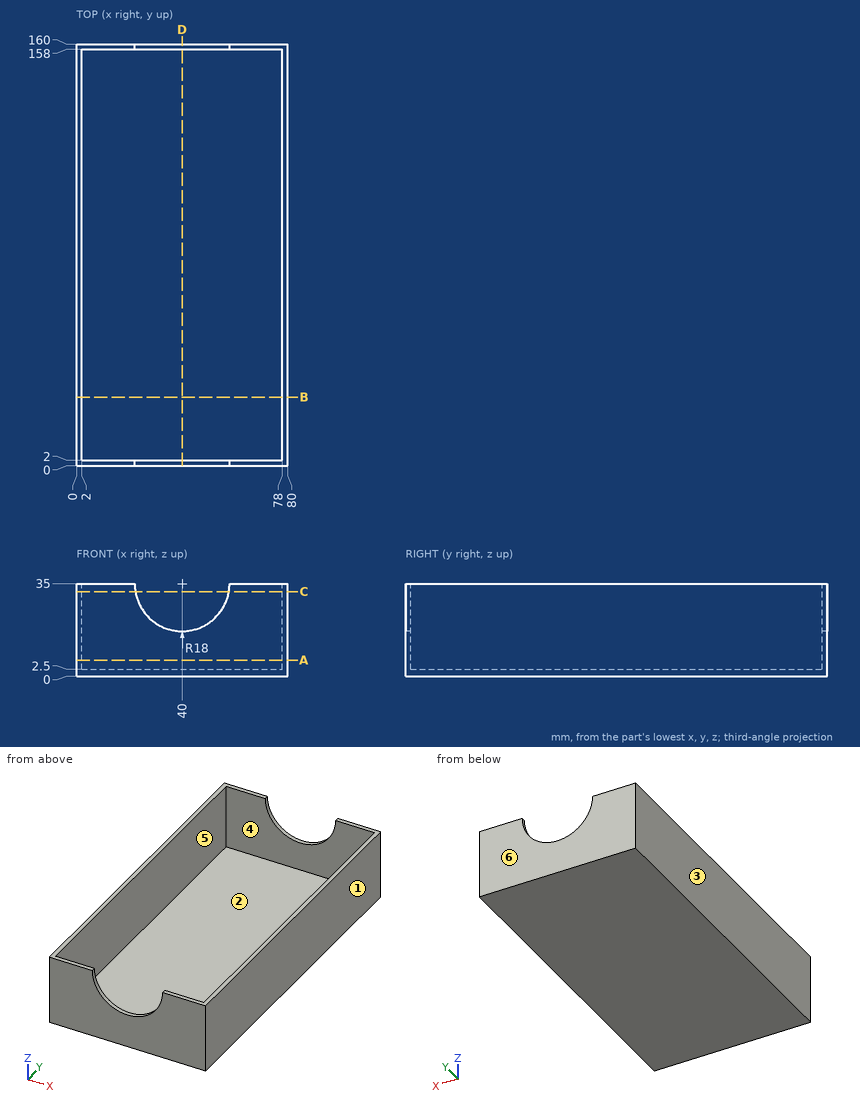
Input: dimensioned drawing with shaded views. Units: mm. Origin: part minimum x, y, z. A direction names the side the tool comes from. Round coordinates to 2 decimals unless told otherwise and drop trailing zeros. Loops run counter-clockwise (first coordinate to the right, second up) from the corner with the lowest first, then second, coordinate; pieces in that order, holes last. Notation, with made-up numbers: (52.25, 4.5) -> (57.25, 4.5) arc R25 cw to (57.25, 39.5) -> close; hole circle Ø8 at (13, 48). An arc over 180 degrees is marked (long way). Answer as a JSON object with one key per item and string values. Group by question number.
Q1. Section query C-C (z = 32). Output: boundary loops of the cut face in (x, y), plus the area to 3 significant figures.
Q2. Section query B-B (y = 26). Output: boundary loops of the cut face in (x, z), plus the area to 3 significant figures.
Q3. Section query D-D (x = 40). Output: boundary loops of the cut face in (y, z), plus the area to 3 significant figures.
Q4. Access query for the marked faces 1 and 2. Directions: +Z, -Z, +X, -X, +Y, -Y. A direction counts if a zero-diameter tool reaches every point of the face in a straight line with its end or side. Return the directions, or none.
Q5. Ray query, line 1 (X direction, y = 84.5, z = 16); line 2 (Y direction, x = 56.5, z = 16); line 3 (Z direction, x = 13, y = 49). Return the intervals inside material, ascending. Write a range as from..to.
Q6. Section query A-A (z = 6). Output: boundary loops of the cut face in (x, y).
Q7. Mould query, pull axis Y, two halves, no side actions, for the marked faces 3, 4, 5 and 6. Classes: pulls with the +Y half, pulls with the -Y half, needs draft (parallel to the pull), parting line crosses it, or undercut.
Completed:
{
 "1": {"outline": "(0, 0) -> (22.25, 0) -> (22.25, 2) -> (2, 2) -> (2, 158) -> (22.25, 158) -> (22.25, 160) -> (0, 160) -> close; (57.75, 0) -> (80, 0) -> (80, 160) -> (57.75, 160) -> (57.75, 158) -> (78, 158) -> (78, 2) -> (57.75, 2) -> close", "area": "802 mm²"},
 "2": {"outline": "(0, 0) -> (80, 0) -> (80, 35) -> (78, 35) -> (78, 2.5) -> (2, 2.5) -> (2, 35) -> (0, 35) -> close", "area": "330 mm²"},
 "3": {"outline": "(0, 0) -> (160, 0) -> (160, 17) -> (158, 17) -> (158, 2.5) -> (2, 2.5) -> (2, 17) -> (0, 17) -> close", "area": "458 mm²"},
 "4": {"face 1": "+Z, -Z, +X, +Y, -Y", "face 2": "+Z"},
 "5": {"line 1": "0..2, 78..80", "line 2": "0..2, 158..160", "line 3": "0..2.5"},
 "6": {"outline": "(0, 0) -> (80, 0) -> (80, 160) -> (0, 160) -> close; hole (2, 2) -> (78, 2) -> (78, 158) -> (2, 158) -> close"},
 "7": {"face 3": "needs draft", "face 4": "undercut", "face 5": "undercut", "face 6": "pulls with the +Y half"}
}
